Read the model definition and answer for the solid it produces. Units are mm, in the model's axes. Coordinates: 2 decimals unless noted, no trailing zeros. Loops run counter-clockwise (first coordinate to the right, second up) from the corner with the lowest first, then second, coordinate; pieces in that order, holes last. Notation, with made-up numbers: (-37.75, 54.5) - (20.25, 54.5) arc R29 ccw to (20.25, 89.5) - close; hole circle Ø8 at (10, 6). An arc over 180 degrees is marked (long way). Use one line per item in the form item = value. Start each with the question number.
1) A cutting plane is placed at C-C (x = 48.5). Give the vertices of the cut face in (y, z).
2) A cutting plane is placed at D-D (z = 0.25). Give the vertices of the cut face in (x, y) (3 decimals), and give its area (3 significant figures).
3) This flat-tipped pin is pushed along its axis until it touches: P1, Ø5.5, axis at x = 93.49, y = -53.98, coming from the -Z side. Where does it stop, or does it pass through?
4) A cutting plane is placed at B-B (y = 107.95). Give the vertices of the cut face in (x, z).
5) A cutting plane is placed at A-A (x = 0). Give the vertices of the cut face in (y, z).
6) Consider line 1 (Y direction, x = 0, z = 0.45); line 2 (X direction, y = -55, z = 0.25); line 3 (Y direction, x = 7.5, z = 1). Determine where each line is inside the solid, lowest interval first.
from build123d import *

# Parameters (mm, degrees)
SKETCH1_R               = 127
BOSS_EXTRUDE1_DEPTH     = 1.5875
F_1_4_CLEARANCE_HOLE1_D = 7.14248
CUT_EXTRUDE1_REACH      = 181.612
SKETCH4_R               = 63.5


with BuildPart() as part:
    # Sketch1 → Boss-Extrude1 (new body)
    with BuildSketch(Plane.XY):
        Circle(SKETCH1_R)
    extrude(amount=BOSS_EXTRUDE1_DEPTH)

    # 1/4 Clearance Hole1 (through all)
    with Locations(Plane.XY.offset(1.5875)):
        with Locations((-93.487442339, 53.975), (0, 107.95), (93.487442339, 53.975), (93.487442339, -53.975), (0, -107.95), (-93.487442339, -53.975)):
            Hole(F_1_4_CLEARANCE_HOLE1_D / 2)

    # Sketch4 → Cut-Extrude1 (cut, up to next)
    with BuildSketch(Plane.XY.offset(1.5875), mode=Mode.PRIVATE) as cut_extrude1_sk1:
        Circle(SKETCH4_R)
    cut_extrude1_tool1 = extrude(cut_extrude1_sk1.sketch, amount=-CUT_EXTRUDE1_REACH, mode=Mode.PRIVATE) & part.part
    add(cut_extrude1_tool1.solids().sort_by_distance((0, 0, 1.5875))[0], mode=Mode.SUBTRACT)


solid = part.part
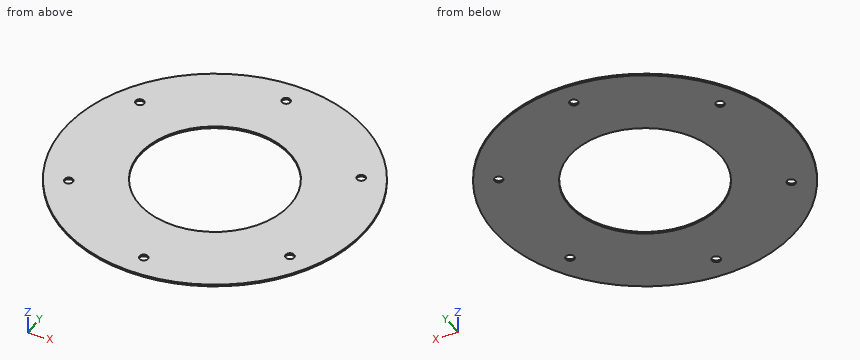
Found:
q1.outline = (-117.37, 0) - (-40.99, 0) - (-40.99, 1.59) - (-117.37, 1.59) - close; (40.99, 0) - (117.37, 0) - (117.37, 1.59) - (40.99, 1.59) - close
q2.outline = circle Ø254 at (0, 0); hole circle Ø7.142 at (-93.487, -53.975); hole circle Ø7.142 at (-93.487, 53.975); hole circle Ø127 at (0, 0); hole circle Ø7.142 at (0, -107.95); hole circle Ø7.142 at (0, 107.95); hole circle Ø7.142 at (93.487, -53.975); hole circle Ø7.142 at (93.487, 53.975)
q2.area = 37,800 mm^2
q3.P1 = through
q4.outline = (-66.9, 0) - (-3.57, 0) - (-3.57, 1.59) - (-66.9, 1.59) - close; (3.57, 0) - (66.9, 0) - (66.9, 1.59) - (3.57, 1.59) - close
q5.outline = (-127, 0) - (-111.52, 0) - (-111.52, 1.59) - (-127, 1.59) - close; (-104.38, 0) - (-63.5, 0) - (-63.5, 1.59) - (-104.38, 1.59) - close; (63.5, 0) - (104.38, 0) - (104.38, 1.59) - (63.5, 1.59) - close; (111.52, 0) - (127, 0) - (127, 1.59) - (111.52, 1.59) - close
q6.line_1 = -127 to -111.52, -104.38 to -63.5, 63.5 to 104.38, 111.52 to 127
q6.line_2 = -114.47 to -96.91, -90.07 to -31.74, 31.74 to 90.07, 96.91 to 114.47
q6.line_3 = -126.78 to -63.06, 63.06 to 126.78
